Check sheet for the modelled part. Datum: model origin and axes. Units: mm. A direction names the side the tool comes from. Coordinates: 2 decimals unless noted, no trailing zeros. Write each loop counter-clockwise with the first axis right and the second up, starting at its lowest first coordinate (ties: lowest second). Pieces come first, ordered by that corner, then holes. Notation, with made-up numbers: (49, 31.25) - (75, 31.25) arc R12 cw to (75, 35.25) - close; hole circle Ø8 at (14, 8). An arc over 180 degrees is marked (long way). Answer as CSV lines item,"result". Start each with the question number.
from build123d import *

# Parameters (mm, degrees)
F1_DEPTH = 5.08
F2_T     = -1.27
F3_R     = 2.54


with BuildPart() as f1:
    # F0 (on Top) → F1 (new body)
    with BuildSketch(Plane.XY):
        with BuildLine():
            ThreePointArc((22.86, 7.62), (21.372102, 11.212102), (17.78, 12.7))
            Line((17.78, 12.7), (-17.78, 12.7))
            ThreePointArc((-17.78, 12.7), (-21.372102, 11.212102), (-22.86, 7.62))
            Line((-22.86, 7.62), (-22.86, -7.62))
            ThreePointArc((-22.86, -7.62), (-21.372102, -11.212102), (-17.78, -12.7))
            Line((-17.78, -12.7), (17.78, -12.7))
            ThreePointArc((17.78, -12.7), (21.372102, -11.212102), (22.86, -7.62))
            Line((22.86, -7.62), (22.86, 7.62))
        make_face()
    extrude(amount=F1_DEPTH)

    # F2
    f2_openings = [f1.faces().sort_by_distance(p)[0] for p in [
        (0, 0, 0),
    ]]
    offset(amount=F2_T, openings=f2_openings)

    # F3
    f3_edges = [f1.edges().sort_by_distance(p)[0] for p in [
        (0, 12.7, 5.08),
    ]]
    fillet(f3_edges, radius=F3_R)


solid = f1.part
(1) Release check for a two-part mould opening along X. For faces 1 (the face through (0.249, -11.976, 4.316)), 2 (the face through (22.86, 0, 1)), 3 (the face through (0, 11.43, 2)), 4 (the face through (-20.444, 10.344, 1.878)) record: pulls with the +X half, pulls with the -X half, needs draft (parallel to the pull), parting line crosses it, or undercut.
(2) Go/stop test with flat-tipped pins: P1, Ø1.5, axis at y = 8, z = 3.5, coming from the -X side; P2, Ø1, axis at x = 13.5, y = -8, coming from the -Z side; P3, Ø1.5, axis at y = -3.5, z = 3.5, coming from the +X side. Record where each tip stops, or that it passes through.
(3) Material ranges on probe 1 along Y at (x, z) = (9.5, 2.45); probe 2 along X at (y, z) = (-6.5, 0.25); probe 3 along Z at (x, y) = (-8, -8), recorded low to high. Write a range as from..to.
(4) Cross-section at A-A on z = 1.7. Record the boundary of the cut face in (x, y), plus the area to 3 significant figures.
(5) Tool access check on faces 5 (the face through (0, 12.7, 1)), 6 (the face through (20.504, 10.284, 1.878)). Record the directions out of +Z, -Z, +X, -X, +Y, -Y that give a thin tool (end or side, any length) a straight path to the whole face; none if there is none.
(6) Cross-section at C-C on y = -7. Record the boundary of the cut face in (x, z).
(7) Cross-section at B-B on x = 15. Record the boundary of the cut face in (y, z).
Checked values:
1,face 1,"needs draft"
1,face 2,"pulls with the +X half"
1,face 3,"undercut"
1,face 4,"undercut"
2,P1,"x = -22.85"
2,P2,"z = 3.81"
2,P3,"x = 22.85"
3,probe 1,"-12.7..-11.43, 11.43..12.7"
3,probe 2,"-22.86..-21.59, 21.59..22.86"
3,probe 3,"3.81..5.08"
4,outline,"(-22.86, -7.62) arc R5.08 ccw to (-17.78, -12.7) - (17.78, -12.7) arc R5.08 ccw to (22.86, -7.62) - (22.86, 7.62) arc R5.08 ccw to (17.78, 12.7) - (-17.78, 12.7) arc R5.08 ccw to (-22.86, 7.62) - close; hole (-21.59, -7.62) arc R3.81 ccw to (-17.78, -11.43) - (17.78, -11.43) arc R3.81 ccw to (21.59, -7.62) - (21.59, 7.62) arc R3.81 ccw to (17.78, 11.43) - (-17.78, 11.43) arc R3.81 ccw to (-21.59, 7.62) - close"
4,area,"165 mm^2"
5,face 5,"+Z, -Z, +X, -X, +Y"
5,face 6,"-Z"
6,outline,"(-22.86, 0) - (-21.59, 0) - (-21.59, 3.81) - (21.59, 3.81) - (21.59, 0) - (22.86, 0) - (22.86, 2.54) arc R2.54 ccw to (20.32, 5.08) - (-20.32, 5.08) arc R2.54 ccw to (-22.86, 2.54) - close"
7,outline,"(-12.7, 0) - (-11.43, 0) - (-11.43, 3.81) - (11.43, 3.81) - (11.43, 0) - (12.7, 0) - (12.7, 2.54) arc R2.54 ccw to (10.16, 5.08) - (-10.16, 5.08) arc R2.54 ccw to (-12.7, 2.54) - close"
